For this review, use the dimensioned drawing (mm, ordinates from the lowest corner) and the shaded views. Coordinates: 2 decimals unless noted, no trailing zeros. Order: outer loops, then holes, each group sorted by start corner. A loop starts at its lowest first (then second) coordinate and runs counter-clockwise, first axis right, second up. Notation, with made-up numbers: (83, 52.25) -> (87, 52.25) arc R14 cw to (87, 75.25) -> close; hole circle Ø6 at (25.5, -12.75). An arc over 180 degrees is marked (long way). Use one line per item in the form item = value. Start each with the question number.
(1) Take a section at C-C (z = 16). State the section outline as (x, y) points, then the cut area to 3 significant figures.
(2) Mouldability with a two-part tool opening along Z and no side actions: class the marked faces 1, 2 and 3 as +Z half, -Z half, draft (parallel to the pull), parting line (faces both ways), or undercut.
(3) Insertion check: pin 1 Ø1.6 at (y, z) = (1.5, 19) entering from +X; pin 2 Ø1.5 at (x, z) = (2.5, 3) entering from +Y; pin 3 Ø1.1 at (x, z) = (1.5, 19.5) entering from -Y. Each pin has a flat end and moves straight along its axis. Give the tip position at first contact, or say it passes through.
(4) Take a section at D-D (x = 2.3). State the section outline as (y, z) points, then the cut area to 3 significant figures.
(5) Take a section at B-B (y = 1.5). State the section outline as (x, z) points, then the cut area to 3 significant figures.
(6) Wall thickness on line 1 along Z through (x, y) = (0.85, 2.7); line 2 along X through (y, z) = (1.6, 3.25); line 3 along Z through (x, y) = (2.8, 0.85): over which ranges is each line inside the solid? List them lowest first.
(7) Take a section at A-A (x = 1.5). State the section outline as (y, z) points.
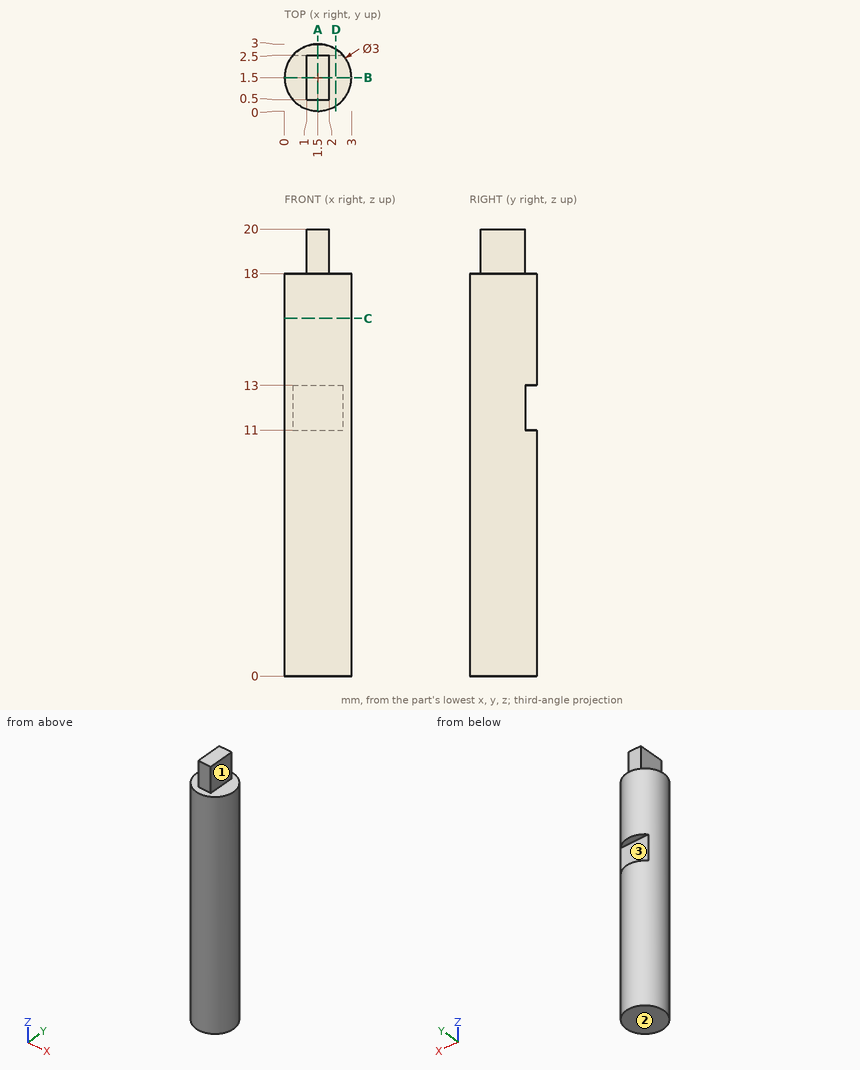
Findings:
q1.outline = circle Ø3 at (1.5, 1.5)
q1.area = 7.07 mm²
q2.face_1 = draft
q2.face_2 = -Z half
q2.face_3 = undercut
q3.pin_1 = 2
q3.pin_2 = 2.98
q3.pin_3 = 0.5
q4.outline = (0.23, 0) -> (2.77, 0) -> (2.77, 11) -> (2.5, 11) -> (2.5, 13) -> (2.77, 13) -> (2.77, 18) -> (0.23, 18) -> close
q4.area = 45.1 mm²
q5.outline = (0, 0) -> (3, 0) -> (3, 18) -> (2, 18) -> (2, 20) -> (1, 20) -> (1, 18) -> (0, 18) -> close
q5.area = 56.0 mm²
q6.line_1 = 0 to 11, 13 to 18
q6.line_2 = 0 to 3
q6.line_3 = 0 to 18
q7.outline = (0, 0) -> (3, 0) -> (3, 11) -> (2.5, 11) -> (2.5, 13) -> (3, 13) -> (3, 18) -> (2.5, 18) -> (2.5, 20) -> (0.5, 20) -> (0.5, 18) -> (0, 18) -> close
